```python
from build123d import *

# Parameters (mm, degrees)
CYLINDER001_R     = 4.05
CYLINDER001_DEPTH = 28
CYLINDER_R        = 6
CYLINDER_DEPTH    = 12
SKETCH_R          = 7
PAD_DEPTH         = 2
CHAMFER_SIZE      = 0.99
CHAMFER001_SIZE   = 1
CHAMFER002_SIZE   = 0.5


with BuildPart() as cilindro001:
    # Cylinder001 → Cylinder001 (new body)
    with BuildSketch(Plane.XY.offset(-1)):
        Circle(CYLINDER001_R)
    extrude(amount=CYLINDER001_DEPTH)


with BuildPart() as chamfer002:
    # Cylinder → Cylinder (new body)
    with BuildSketch(Plane.XY):
        Circle(CYLINDER_R)
    extrude(amount=CYLINDER_DEPTH)

    # Sketch → Pad (new body)
    with BuildSketch(Plane.XY.offset(12)):
        Circle(SKETCH_R)
    extrude(amount=PAD_DEPTH)

    # Cut: cut Cilindro001
    add(cilindro001.part, mode=Mode.SUBTRACT)

    # Chamfer
    chamfer_edges = [chamfer002.edges().sort_by_distance(p)[0] for p in [
        (-6, 0, 12),
    ]]
    chamfer(chamfer_edges, length=CHAMFER_SIZE)

    # Chamfer001
    chamfer001_edges = [chamfer002.edges().sort_by_distance(p)[0] for p in [
        (-6, 0, 0),
    ]]
    chamfer(chamfer001_edges, length=CHAMFER001_SIZE)

    # Chamfer002
    chamfer002_edges = [chamfer002.edges().sort_by_distance(p)[0] for p in [
        (-4.05, 0, 14),
    ]]
    chamfer(chamfer002_edges, length=CHAMFER002_SIZE)


solid = chamfer002.part
```
For this review, take the finished solid that the model builds, in its own axes (mm). A direction names the side the tool comes from. Round coordinates to 2 decimals unless told otherwise and drop trailing zeros. Write each loop counter-clockwise with the first axis right and the second up, starting at its lowest first coordinate (ties: lowest second). Pieces come first, ordered by that corner, then holes. Notation, with made-up numbers: (13.25, 47.5) -> (33.25, 47.5) arc R19 ccw to (33.25, 62.5) -> close; hole circle Ø1 at (-13, -9.75). An arc over 180 degrees is marked (long way). Use one line per item in the form item = value.
1) Tool access review of faces 1 (the flat face through (2, -4, 0)), 2 (the cylindrical face through (-6, 0, 6)): name each direction out of +Z, -Z, +X, -X, +Y, -Y from which nothing blocks a thin tool from reaching the whole face with its end or side.
Found:
face_1 = -Z, +X, -X, +Y, -Y
face_2 = -Z
2) To check wall thickness, follow L1, parallel to Y at x = 0, z = 12.25; L2, parallel to Y at x = 0, z = 6.25; L3, parallel to X at y = -2, z = 5. State the ranges of each line that lie inside material, in increasing order. Write a range as from..to.
Found:
L1 = -7..-4.05, 4.05..7
L2 = -6..-4.05, 4.05..6
L3 = -5.66..-3.52, 3.52..5.66
3) Clearance check with flat-ended pins moving along their axes: pin 1 (5 mm diameter, centred on x = 0, y = 0, fed in from +Z); pin 2 (1.5 mm diameter, centred on y = -5.5, z = 2, fed in from -X); pin 3 (1.5 mm diameter, centred on y = -4.5, z = 7, fed in from +X); pin 4 (3 mm diameter, centred on y = -3.5, z = 9.5, fed in from -X). State where each tip first meets the part, or that it passes through.
Found:
pin_1 = through
pin_2 = -3.67
pin_3 = 4.68
pin_4 = -5.66
4) Mouldability with a two-part tool opening along Y and no side actions: class faces 3 (the cylindrical face through (6.466, -2.681, 12.986)), 4 (the cylindrical face through (-0.878, -3.954, 6.656)), 5 (the flat face through (0, -5, 14)) as +Y half, -Y half, draft (parallel to the pull), parting line (faces both ways), or undercut.
Found:
face_3 = parting line
face_4 = undercut
face_5 = draft
5) Take a section at C-C, the plane z = 7. Write out the cut boundary in (x, y), and give its area (3 significant figures).
Found:
outline = circle Ø12 at (0, 0); hole circle Ø8.1 at (0, 0)
area = 61.6 mm2
